Check sheet for the modelled part. Datum: model origin and axes. Units: mm. A direction names the side the tool comes from. Round coordinates to 2 decimals unless told otherwise and drop trailing zeros. Order: outer loops, then holes, each group sorted by start corner. A loop starts at its lowest first (then second) coordinate and runs counter-clockwise, first axis right, second up. Notation, with made-up numbers: (81.25, 1.25) -> (93.25, 1.25) arc R22 cw to (93.25, 22.25) -> close; hole circle Ø6 at (-22.75, 73.5). An arc over 180 degrees is marked (long way). Answer in a Markdown table with one row per item.
```python
from build123d import *

# Parameters (mm, degrees)
IZIM1_R                     = 9
Y_KSEKLIK_EKSTR_ZYON1_DEPTH = 51.8
IZIM2_R                     = 3.5
Y_KSEKLIK_EKSTR_ZYON2_DEPTH = 8
Y_KSEKLIK_EKSTR_ZYON2_TAPER = 5
Y_KSEKLIK_EKSTR_ZYON3_DEPTH = 6
LPATTERN1_COUNT             = 2
LPATTERN1_PITCH             = 15


with BuildPart() as part:
    # Çizim1 → Yükseklik-Ekstrüzyon1 (new body)
    with BuildSketch(Plane.XY):
        with Locations(Location((0, 0, 0), (0, 0, 180))):
            Circle(IZIM1_R)
    extrude(amount=Y_KSEKLIK_EKSTR_ZYON1_DEPTH)

    # Çizim2 → Yükseklik-Ekstrüzyon2 (add)
    with BuildSketch(Plane.XY.offset(51.8)):
        with Locations((2.961323267, 2.878406216)):
            Circle(IZIM2_R)
    extrude(amount=Y_KSEKLIK_EKSTR_ZYON2_DEPTH, taper=Y_KSEKLIK_EKSTR_ZYON2_TAPER)

    # Çizim6 → Yükseklik-Ekstrüzyon3 (add)
    with BuildSketch(Plane(origin=(0, 0, 6.81), x_dir=(-1, 0, 0), z_dir=(0, 0, -1))):
        Polygon((6.062177826, 10.5), (-6.062177826, 10.5), (-12.124355653, 0), (-6.062177826, -10.5), (6.062177826, -10.5), (12.124355653, 0), align=None)
    y_kseklik_ekstr_zyon3 = extrude(amount=-Y_KSEKLIK_EKSTR_ZYON3_DEPTH)

    # LPattern1: Yükseklik-Ekstrüzyon3 ×2
    with Locations(*[(0, 0, i * LPATTERN1_PITCH) for i in range(1, LPATTERN1_COUNT)]):
        add(y_kseklik_ekstr_zyon3)


solid = part.part
```
(1) Depth check by flat-ended pin: pin 1 Ø8 at (x, y) = (1, -6) entering from +Z; pin 2 Ø5 at (x, z) = (9, 39) entering from +Y; pin 3 Ø5 at (x, z) = (2.5, 48) entering from +Y. Enter the tip coordinate at first touch or a pass-through.
Solutions:
| item | result |
|---|---|
| pin 1 | z = 51.8 |
| pin 2 | y = 6.22 |
| pin 3 | y = 9 |
(2) Section check C-C on x = -4.5. Record the boundary of the cut face in (y, z).
Solutions:
| item | result |
|---|---|
| outline | (-10.5, 6.81) -> (-7.79, 6.81) -> (-7.79, 0) -> (7.79, 0) -> (7.79, 6.81) -> (10.5, 6.81) -> (10.5, 12.81) -> (7.79, 12.81) -> (7.79, 21.81) -> (10.5, 21.81) -> (10.5, 27.81) -> (7.79, 27.81) -> (7.79, 51.8) -> (-7.79, 51.8) -> (-7.79, 27.81) -> (-10.5, 27.81) -> (-10.5, 21.81) -> (-7.79, 21.81) -> (-7.79, 12.81) -> (-10.5, 12.81) -> close |
(3) Section check D-D on z = 46.5. Record the boundary of the cut face in (x, y).
Solutions:
| item | result |
|---|---|
| outline | circle Ø18 at (0, 0) |
(4) Draft check along Z on faces 4 (the flat face through (0, 0, 0)), 5 (the flat face through (-9.051, -5.324, 24.768)), 6 (the cylindrical face through (6.633, -6.083, 17.247)). Enter one of: pulls with the +Z half, pulls with the -Z half, needs draft (parallel to the pull), parting line crosses it, or undercut.
Solutions:
| item | result |
|---|---|
| face 4 | pulls with the -Z half |
| face 5 | needs draft |
| face 6 | undercut |
(5) Tool access check on faces 1 (the flat face through (0, 10.5, 10)), 2 (the flat face through (3, 9, 27.81)), 3 (the cylindrical face through (6.633, -6.083, 3.357)). Record the directions out of +Z, -Z, +X, -X, +Y, -Y that give a thin tool (end or side, any length) a straight path to the whole face; none if there is none.
Solutions:
| item | result |
|---|---|
| face 1 | +Z, -Z, +X, -X, +Y |
| face 2 | +Z |
| face 3 | -Z |
(6) Section check B-B on y = -4.75. Record the boundary of the cut face in (x, z).
Solutions:
| item | result |
|---|---|
| outline | (-9.38, 6.81) -> (-7.64, 6.81) -> (-7.64, 0) -> (7.64, 0) -> (7.64, 6.81) -> (9.38, 6.81) -> (9.38, 12.81) -> (7.64, 12.81) -> (7.64, 21.81) -> (9.38, 21.81) -> (9.38, 27.81) -> (7.64, 27.81) -> (7.64, 51.8) -> (-7.64, 51.8) -> (-7.64, 27.81) -> (-9.38, 27.81) -> (-9.38, 21.81) -> (-7.64, 21.81) -> (-7.64, 12.81) -> (-9.38, 12.81) -> close |
(7) Section check A-A on z = 24.5. Record the boundary of the cut face in (x, y).
Solutions:
| item | result |
|---|---|
| outline | (-12.12, 0) -> (-6.06, -10.5) -> (6.06, -10.5) -> (12.12, 0) -> (6.06, 10.5) -> (-6.06, 10.5) -> close |
(8) Scan lines: probe 1 along Z at (x, y) = (6.25, -8.25); probe 2 along Z at (x, y) = (-0.25, -6); probe 3 along X at (y, z) = (-5.5, 46). Record each from-to range of solid material in increasing order. Write a range as from..to.
Solutions:
| item | result |
|---|---|
| probe 1 | 6.81..12.81, 21.81..27.81 |
| probe 2 | 0..51.8 |
| probe 3 | -7.12..7.12 |
